Geometry check sheet. Reference: the model listing, model coordinates, mm. A direction names the side the tool comes from. Coordinates: 2 decimals unless noted, no trailing zeros. Write each loop counter-clockwise with the first axis right and the second up, starting at its lowest first coordinate (ties: lowest second). Pieces come first, ordered by that corner, then holes. Notation, with made-up numbers: (57, 40.5) -> (62, 40.5) arc R29 ccw to (62, 66.5) -> close; hole circle Ø4 at (71, -21.75). An arc over 180 degrees is marked (long way). Use a Markdown table: item, result.
```python
from build123d import *

# Parameters (mm, degrees)
SKETCH1_R           = 1.655864604
BOSS_EXTRUDE1_DEPTH = 3
SKETCH2_W           = 20
SKETCH2_H           = 25.399582392
SKETCH2_R           = 1.655864604
BOSS_EXTRUDE2_DEPTH = 16
SKETCH3_W           = 14
SKETCH3_H           = 30.433665038
CUT_EXTRUDE1_DEPTH  = 12
FILLET1_R           = 3
SKETCH4_R           = 3.655864604
CUT_EXTRUDE2_DEPTH  = 3


with BuildPart() as part:
    # Sketch1 → Boss-Extrude1 (new body)
    with BuildSketch(Plane(origin=(0, 0, 0), x_dir=(1, 0, 0), z_dir=(0, 1, 0))):
        with BuildLine():
            Line((-72.391156815, 44.965534322), (-72.391156815, -60.735574691))
            add(Edge.make_bspline(
                [(-72.391156815, -60.735574691), (-72.391156815, -61.992108225), (-72.131767652, -63.841263996), (-71.193134075, -66.331246924), (-70.115754462, -68.193455339), (-68.602916824, -69.990155744), (-66.871043197, -71.356237465), (-65.167773111, -72.264127558), (-63.671954883, -72.82246992), (-62.083143976, -73.170982974), (-60.950569944, -73.258988683), (-60.391156815, -73.258988683)],
                knots=[0, 0, 0, 0, 0.25, 0.375, 0.5, 0.625, 0.75, 0.8125, 0.875, 0.9375, 1, 1, 1, 1], degree=3))
            Line((-60.391156815, -73.258988683), (59.608843185, -73.258988683))
            add(Edge.make_bspline(
                [(59.608843185, -73.258988683), (60.161825687, -73.258988683), (61.27919765, -73.173963171), (62.86030745, -72.830650997), (64.348694962, -72.279953513), (66.061771772, -71.375336188), (67.804355953, -70.006238159), (69.822626853, -67.61666824), (71.258952654, -64.479060557), (71.608843185, -61.999282855), (71.608843185, -60.735574691)],
                knots=[0, 0, 0, 0, 0.0625, 0.125, 0.1875, 0.25, 0.375, 0.5, 0.75, 1, 1, 1, 1], degree=3))
            Line((71.608843185, -60.735574691), (71.608843185, 44.965534322))
            ThreePointArc((71.608843185, 44.965534322), (68.094124559, 53.450815696), (59.608843185, 56.965534322))
            Line((59.608843185, 56.965534322), (-60.391156815, 56.965534322))
            ThreePointArc((-60.391156815, 56.965534322), (-68.876438189, 53.450815696), (-72.391156815, 44.965534322))
        make_face()
        with Locations((0.208651948, 24.377980521)):
            Circle(SKETCH1_R, mode=Mode.SUBTRACT)
        with Locations((-0.01971378, 9.762573941)):
            Circle(SKETCH1_R, mode=Mode.SUBTRACT)
    extrude(amount=BOSS_EXTRUDE1_DEPTH)

    # Sketch2 → Boss-Extrude2 (add)
    with BuildSketch(Plane(origin=(0, 3, 0), x_dir=(1, 0, 0), z_dir=(0, 1, 0))):
        with Locations((0.161550821, 16.648607969)):
            Rectangle(SKETCH2_W, SKETCH2_H)
        with Locations((-0.01971378, 9.762573941)):
            Circle(SKETCH2_R, mode=Mode.SUBTRACT)
        with Locations((0.208651948, 24.377980521)):
            Circle(SKETCH2_R, mode=Mode.SUBTRACT)
    extrude(amount=BOSS_EXTRUDE2_DEPTH)

    # Sketch3 → Cut-Extrude1 (cut)
    with BuildSketch(Plane(origin=(0, 19, 0), x_dir=(1, 0, 0), z_dir=(0, 1, 0))):
        with Locations((0.269010393, 16.661700324)):
            Rectangle(SKETCH3_W, SKETCH3_H)
    extrude(amount=-CUT_EXTRUDE1_DEPTH, mode=Mode.SUBTRACT)

    # Fillet1
    fillet1_edges = [part.edges().sort_by_distance(p)[0] for p in [
        (-9.838449179, 3, -16.648607969),
        (10.161550821, 3, -16.648607969),
    ]]
    fillet(fillet1_edges, radius=FILLET1_R)

    # Sketch4 → Cut-Extrude2 (cut)
    with BuildSketch(Plane.XZ):
        with Locations((-0.01971378, -9.762573941)):
            Circle(SKETCH4_R)
        with Locations((0.208651948, -24.377980521)):
            Circle(SKETCH4_R)
    extrude(amount=-CUT_EXTRUDE2_DEPTH, mode=Mode.SUBTRACT)


solid = part.part
```
Item 1: Section check A-A on y = 15.5. Record the boundary of the cut face in (x, z), then the cut area to 3 significant figures.
Answer block:
| item | result |
|---|---|
| outline | (-9.84, -29.35) -> (-6.73, -29.35) -> (-6.73, -3.95) -> (-9.84, -3.95) -> close; (7.27, -29.35) -> (10.16, -29.35) -> (10.16, -3.95) -> (7.27, -3.95) -> close |
| area | 152 mm^2 |
Item 2: Mould release check, pull along X, two halves, no side actions. Record for faces 5 (the flat face through (-9.838, 12, -16)), 6 (the flat face through (1.1, 6.8, -3.949)), 7 (the flat face through (2, 3, -11)): +X half, -X half, draft (parallel to the pull), parting line (faces both ways), or undercut.
Answer block:
| item | result |
|---|---|
| face 5 | -X half |
| face 6 | draft |
| face 7 | undercut |
Item 3: Thickness scan on L1, parallel to Y at x = -40, z = 5; L2, parallel to Z at x = 8.5, y = 17. Record the ranges inside material, lowest first. Write a range as [from, to].
Answer block:
| item | result |
|---|---|
| L1 | y = [0, 3] |
| L2 | z = [-29.35, -3.95] |
Item 4: Section check B-B on x = -44. Record the boundary of the cut face in (y, z).
Answer block:
| item | result |
|---|---|
| outline | (0, -56.97) -> (3, -56.97) -> (3, 73.26) -> (0, 73.26) -> close |
Item 5: Depth check by flat-ended pin: P1, Ø4, axis at x = 2, z = -22.5, coming from the +Y side; P2, Ø8, axis at x = 5, y = 7.5, coming from the +Z side; P3, Ø4, axis at y = 13.5, z = -19, coming from the -X side. Enter the tip coordinate at first touch or a pass-through.
Answer block:
| item | result |
|---|---|
| P1 | stops at y = 7 |
| P2 | stops at z = -3.95 |
| P3 | stops at x = -9.84 |
Item 6: Tool access check on faces 1 (the flat face through (7.269, 13, -16)), 2 (the flat face through (10.162, 12, -16)), 3 (the flat face through (2, 3, -25)), 4 (the flat face through (1.1, 6.8, -29.348)). Record the directions out of +Z, -Z, +X, -X, +Y, -Y that give a thin tool (end or side, any length) a straight path to the whole face; none if there is none.
Answer block:
| item | result |
|---|---|
| face 1 | +Z, -Z, +Y |
| face 2 | +Z, -Z, +X, +Y |
| face 3 | -Y |
| face 4 | -Z, +X, -X, +Y |
Item 7: Section check C-C on z = 39. Record the boundary of the cut face in (x, y), then the cut area to 3 significant figures.
Answer block:
| item | result |
|---|---|
| outline | (-72.39, 0) -> (71.61, 0) -> (71.61, 3) -> (-72.39, 3) -> close |
| area | 432 mm^2 |
